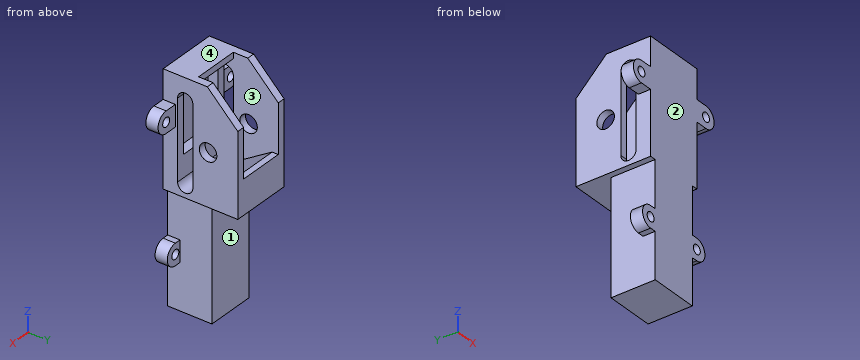
```python
from build123d import *

# Parameters (mm, degrees)
SKETCH1_W               = 16
SKETCH1_H               = 74.5
BOSS_EXTRUDE1_DEPTH     = 14.5
SKETCH2_R               = 1.5
BOSS_EXTRUDE2_DEPTH     = 4
SKETCH3_W               = 2
SKETCH3_H               = 37.25
BOSS_EXTRUDE3_DEPTH     = 14.5
SKETCH4_R               = 1.5
BOSS_EXTRUDE4_DEPTH     = 4
CUT_EXTRUDE1_DEPTH      = 49.487529582
SKETCH7_W               = 20
SKETCH7_H               = 37.25
BOSS_EXTRUDE5_DEPTH     = 10
SKETCH8_W               = 7.5
SKETCH8_H               = 26
SKETCH8_W_2             = 7.486605722
CUT_EXTRUDE2_DEPTH      = 23
SKETCH10_W              = 14.986605722
SKETCH10_H              = 2
BOSS_EXTRUDE6_DEPTH     = 13
CUT_EXTRUDE3_DEPTH      = 14.986605722
SKETCH13_W              = 14.986605722
SKETCH13_H              = 0.75
CUT_EXTRUDE4_DEPTH      = 1
SKETCH14_R              = 2.875
CUT_EXTRUDE5_DEPTH      = 53.354947474
CUT_EXTRUDE6_DEPTH      = 52.088800387
CUT_EXTRUDE6_DEPTH_BACK = 52.088800387
SKETCH16_W              = 14.986605722
SKETCH16_H              = 2
CUT_EXTRUDE7_DEPTH      = 4.75


with BuildPart() as part:
    # Sketch1 → Boss-Extrude1 (new body)
    with BuildSketch(Plane(origin=(0, 0, 0), x_dir=(1, 0, 0), z_dir=(0, 1, 0))):
        Rectangle(SKETCH1_W, SKETCH1_H)
    extrude(amount=BOSS_EXTRUDE1_DEPTH)

    # Sketch2 → Boss-Extrude2 (add)
    with BuildSketch(Plane(origin=(0, 0, 0), x_dir=(-1, 0, 0), z_dir=(0, -1, 0))):
        with BuildLine():
            Line((8, 22.25), (8, 18.75))
            Line((8, 18.75), (8, 15.25))
            Line((8, 15.25), (9.975, 15.25))
            ThreePointArc((9.975, 15.25), (13.475, 18.75), (9.975, 22.25))
            Line((9.975, 22.25), (8, 22.25))
        make_face()
        with Locations(Location((9.975, 18.75, 0), (0, 0, 90))):
            Circle(SKETCH2_R, mode=Mode.SUBTRACT)
    boss_extrude2 = extrude(amount=-BOSS_EXTRUDE2_DEPTH)

    # Mirror1: Boss-Extrude2 across plane
    add(boss_extrude2.mirror(Plane(origin=(0, 0, 0), x_dir=(0, 0, 1), z_dir=(1, 0, 0))))

    # Sketch3 → Boss-Extrude3 (add)
    with BuildSketch(Plane(origin=(0, 0, 0), x_dir=(-1, 0, 0), z_dir=(0, -1, 0))):
        with Locations((9, -18.625)):
            Rectangle(SKETCH3_W, SKETCH3_H)
        with Locations((-9, -18.625)):
            Rectangle(SKETCH3_W, SKETCH3_H)
    extrude(amount=-BOSS_EXTRUDE3_DEPTH)

    # Sketch4 → Boss-Extrude4 (add)
    with BuildSketch(Plane(origin=(0, 0, 0), x_dir=(-1, 0, 0), z_dir=(0, -1, 0))):
        with BuildLine():
            Line((10, -20.74), (10, -27.74))
            Line((10, -27.74), (13.945, -27.74))
            ThreePointArc((13.945, -27.74), (17.445, -24.24), (13.945, -20.74))
            Line((13.945, -20.74), (10, -20.74))
        make_face()
        with Locations(Location((13.945, -24.24, 0), (0, 0, 90))):
            Circle(SKETCH4_R, mode=Mode.SUBTRACT)
    boss_extrude4 = extrude(amount=-BOSS_EXTRUDE4_DEPTH)

    # Mirror4: Boss-Extrude4 across plane
    add(boss_extrude4.mirror(Plane(origin=(0, 0, 0), x_dir=(0, 0, 1), z_dir=(1, 0, 0))))

    # Sketch5 → Cut-Extrude1 (cut, through all)
    with BuildSketch(Plane(origin=(10, 0, 0), x_dir=(0, 0, -1), z_dir=(1, 0, 0))):
        with BuildLine():
            Line((-4, 9.75), (-30, 9.75))
            ThreePointArc((-30, 9.75), (-32.5, 7.25), (-30, 4.75))
            Line((-30, 4.75), (-4, 4.75))
            ThreePointArc((-4, 4.75), (-1.5, 7.25), (-4, 9.75))
        make_face()
    extrude(amount=-CUT_EXTRUDE1_DEPTH, mode=Mode.SUBTRACT)

    # Sketch7 → Boss-Extrude5 (add)
    with BuildSketch(Plane(origin=(0, 14.5, 0), x_dir=(1, 0, 0), z_dir=(0, 1, 0))):
        with Locations((0, -18.625)):
            Rectangle(SKETCH7_W, SKETCH7_H)
    extrude(amount=BOSS_EXTRUDE5_DEPTH)

    # Sketch8 → Cut-Extrude2 (cut)
    with BuildSketch(Plane(origin=(0, 24.5, 0), x_dir=(1, 0, 0), z_dir=(0, 1, 0))):
        with Locations((3.75, -24.25)):
            Rectangle(SKETCH8_W, SKETCH8_H)
        with Locations((-3.743302861, -24.25)):
            Rectangle(SKETCH8_W_2, SKETCH8_H)
    extrude(amount=-CUT_EXTRUDE2_DEPTH, mode=Mode.SUBTRACT)

    # Sketch10 → Boss-Extrude6 (add)
    with BuildSketch(Plane(origin=(0, 1.5, 0), x_dir=(1, 0, 0), z_dir=(0, 1, 0))):
        with Locations((0.006697139, -36.25)):
            Rectangle(SKETCH10_W, SKETCH10_H)
    extrude(amount=BOSS_EXTRUDE6_DEPTH)

    # Sketch12 → Cut-Extrude3 (cut)
    with BuildSketch(Plane.ZY.offset(-7.5)):
        Polygon((11.25, 9.75), (11.25, 22.5), (3.25, 9.75), align=None)
    extrude(amount=CUT_EXTRUDE3_DEPTH, mode=Mode.SUBTRACT)

    # Sketch13 → Cut-Extrude4 (cut)
    with BuildSketch(Plane(origin=(0, 9.75, 0), x_dir=(1, 0, 0), z_dir=(0, 1, 0))):
        with Locations((0.006697139, -3.625)):
            Rectangle(SKETCH13_W, SKETCH13_H)
    extrude(amount=-CUT_EXTRUDE4_DEPTH, mode=Mode.SUBTRACT)

    # Sketch14 → Cut-Extrude5 (cut, through all)
    with BuildSketch(Plane(origin=(10, 0, 0), x_dir=(0, 0, -1), z_dir=(1, 0, 0))):
        with Locations((-17, 14.75)):
            Circle(SKETCH14_R)
    extrude(amount=-CUT_EXTRUDE5_DEPTH, mode=Mode.SUBTRACT)

    # Sketch15 → Cut-Extrude6 (cut, two sides: drawn at the far end of the back side and taken through both)
    with BuildSketch(Plane.ZY.offset(-7.5).offset(-CUT_EXTRUDE6_DEPTH_BACK)):
        Polygon((37.25, 14.5), (37.25, 24.5), (27.25, 24.5), align=None)
    extrude(amount=CUT_EXTRUDE6_DEPTH + CUT_EXTRUDE6_DEPTH_BACK, mode=Mode.SUBTRACT)

    # Sketch16 → Cut-Extrude7 (cut)
    with BuildSketch(Plane(origin=(0, 14.5, 0), x_dir=(1, 0, 0), z_dir=(0, 1, 0))):
        with Locations((0.006697139, -36.25)):
            Rectangle(SKETCH16_W, SKETCH16_H)
    extrude(amount=-CUT_EXTRUDE7_DEPTH, mode=Mode.SUBTRACT)


solid = part.part
```
The listing builds one solid part. Answer for the finished solid, in the listing's coordinates (mm). Face numbers are marked on the shaded views. A direction names the side the tool comes from. Coordinates: 2 decimals unless noted, no trailing zeros. Loops run counter-clockwise (first coordinate to the right, second up) from the corner with the lowest first, then second, coordinate; pieces in that order, holes last. Notation, with made-up numbers: (-24.75, 74.5) -> (6.25, 74.5) arc R22 cw to (6.25, 95.5) -> close; hole circle Ø10 at (62.5, 58). An arc over 180 degrees is marked (long way). Use one line per item in the form item = value. Start each with the question number.
Item 1: Consider L1, parallel to X at y = 2.15, z = -18.75 (3 decimals); L2, parallel to Y at x = 9.1, z = 17 (3 decimals); L3, parallel to X at y = 3, z = 24.24 (3 decimals). Determine where each line is inside the solid, lowest interval first. Write a range as [from, to].
Item 2: Flat-ended cylindrical pins translate along their axes: pin 1 Ø5 at (y, z) = (18, 27) entering from +X; pin 2 Ø1.6 at (x, z) = (0.5, 36.5) entering from +Y; pin 3 Ø1.3 at (x, z) = (-9, 17.5) entering from -Y; pin 4 Ø1.6 at (x, y) = (-0.5, 23.5) entering from +Z. Find the tip coordinate at first contact, or state that the pin passes through.
Item 3: A tool of negligible diameter and unlimited length cuts with its end or side. For the marked faces 1 and 2, from which of +Z, -Z, +X, -X, +Y, -Y can it reach the whole face along a straight path? Write none if from no direction.
Item 4: The part is cut by section C-C on z = 17. Determine the outline of the cut face in (x, y) (3 decimals), then the cut area to 3 significant figures.
Item 5: The part is cut by section A-A on z = 29. Determine the outline of the cut face in (x, y).
Item 6: The part is cut by section D-D on x = -3. Determine the outline of the cut face in (y, z), then the cut area to 3 significant figures.
Item 7: The part is cut by section B-B on y = 3.25. Count the separate pieces of the cut face and the enclosed holes in it, then the cut area to 3 significant figures.
Item 8: The mould has two halves that part along X. Classify the marked faces 3 and 4: released by +X, released by -X, zero draft, split by the parting line, or undercut.
Answer key:
q1.L1 = [-13.475, -11.475], [-8.475, 8.475], [11.475, 13.475]
q1.L2 = [0, 4.75], [9.75, 11.875], [17.625, 24.5]
q1.L3 = [-17.445, -15.445], [-12.445, -7.487], [7.5, 12.445], [15.445, 17.445]
q2.pin_1 = 10
q2.pin_2 = 9.75
q2.pin_3 = 0
q2.pin_4 = 11.25
q3.face_1 = -Z, +X, -X, +Y
q3.face_2 = +Z, -Z, +X, -X, -Y
q4.outline = (-10, 0) -> (10, 0) -> (10, 4.75) -> (7.5, 4.75) -> (7.5, 1.5) -> (-7.487, 1.5) -> (-7.487, 4.75) -> (-10, 4.75) -> close; (-10, 9.75) -> (-7.487, 9.75) -> (-7.487, 11.875) -> (-10, 11.875) -> close; (-10, 17.625) -> (-7.487, 17.625) -> (-7.487, 24.5) -> (-10, 24.5) -> close; (7.5, 9.75) -> (10, 9.75) -> (10, 11.875) -> (7.5, 11.875) -> close; (7.5, 17.625) -> (10, 17.625) -> (10, 24.5) -> (7.5, 24.5) -> close
q4.area = 91.4 mm2
q5.outline = (-10, 0) -> (10, 0) -> (10, 4.75) -> (7.5, 4.75) -> (7.5, 1.5) -> (-7.49, 1.5) -> (-7.49, 4.75) -> (-10, 4.75) -> close; (-10, 9.75) -> (-7.49, 9.75) -> (-7.49, 22.75) -> (-10, 22.75) -> close; (7.5, 9.75) -> (10, 9.75) -> (10, 22.75) -> (7.5, 22.75) -> close
q6.outline = (0, -37.25) -> (14.5, -37.25) -> (14.5, 0) -> (24.5, 0) -> (24.5, 11.25) -> (22.5, 11.25) -> (9.75, 3.25) -> (9.63, 3.25) arc R2.5 cw to (4.75, 4) -> (4.75, 11.25) -> (1.5, 11.25) -> (1.5, 35.25) -> (9.75, 35.25) -> (9.75, 37.25) -> (0, 37.25) -> close
q6.area = 774 mm2
q7.separate_pieces = 1
q7.enclosed_holes = 5
q7.area = 1,110 mm2
q8.face_3 = undercut
q8.face_4 = zero draft
